Check sheet for the modelled part. Datum: model origin and axes. Units: mm. Give positions to 0.01 mm unless a question says otherwise; leave off trailing zeros. Loops run counter-clockwise (first coordinate to the right, second up) from the corner with the lowest first, then second, coordinate; pieces in that order, holes last. Notation, with made-up numbers: (-8.75, 55.5) -> (22.25, 55.5) arc R18 cw to (22.25, 68.5) -> close; hole circle Ø10 at (20.5, 16). An arc over 180 degrees is marked (long way). Write each question's results on one line, items separated by ' | '. Start each with the question number.
1. Cross-section at B-B on y = 4. Record the boundary of the cut face in (x, z), and give its area (3 significant figures).
2. Cross-section at D-D on z = 2.1. Count the separate pieces of the cut face and the enclosed holes in it, and give its area (3 significant figures).
3. Cross-section at A-A on x = -0.5. Record the boundary of the cut face in (y, z).
4. Cross-section at C-C on x = -48. Record the boundary of the cut face in (y, z), and give its area (3 significant figures).
5. Gauge pin test, flat ends, axial feed: pin 1 Ø2.5 at (x, z) = (-18, 3) entering from +Y; pin 2 Ø3 at (y, z) = (18.5, 0.5) entering from -X; pin 3 Ø2.5 at (x, z) = (-105.5, 3) entering from +Y; pin 4 Ø4.5 at (x, y) = (51.5, 4) entering from +Z. Record the tip position at first contact, or that the pin passes through.
6. Material ranges on L1, parallel to Y at x = 25.5, z = 3.75; L2, parallel to Y at x = -27.5, z = 2.1; L3, parallel to X at y = 48, z = 2.8, recorded low to high. Write a range as from..to.
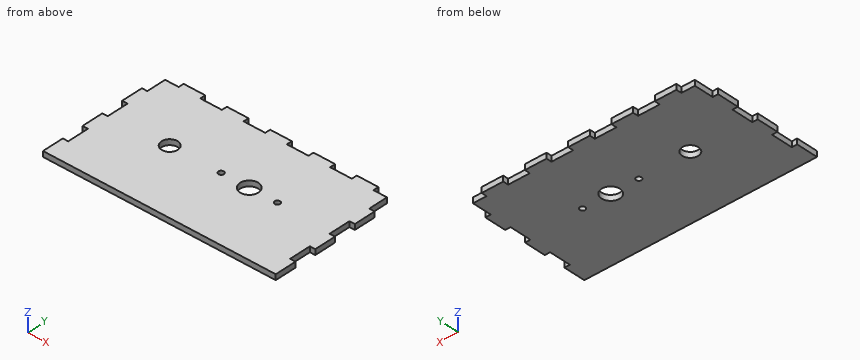
from build123d import *

# Parameters (mm, degrees)
SKETCH_1_W               = 205
SKETCH_1_H               = 118
SKETCH_1_R               = 8.5
SKETCH_1_R_2             = 7.5
SKETCH_1_R_3             = 2.5
EXTRUDE_1_DEPTH          = 5
SKETCH_2_W               = 5
SKETCH_2_H               = 20
EXTRUDE_2_DEPTH          = 5
PATTERN_LINEAR_2_COUNT   = 3
PATTERN_LINEAR_2_PITCH   = 40
MIRROR_2_COPY_1_SKETCH_W = 5
MIRROR_2_COPY_1_SKETCH_H = 20
MIRROR_2_COPY_1_DEPTH    = 5
MIRROR_2_COPY_2_SKETCH_W = 5
MIRROR_2_COPY_2_SKETCH_H = 20
MIRROR_2_COPY_2_DEPTH    = 5
SKETCH_3_W               = 20
SKETCH_3_H               = 5
EXTRUDE_3_DEPTH          = 5
PATTERN_LINEAR_3_COUNT   = 3
PATTERN_LINEAR_3_PITCH   = 40
PATTERN_LINEAR_4_COUNT   = 3
PATTERN_LINEAR_4_PITCH   = 40


with BuildPart() as part:
    # 스케치1 → 보스-돌출1 (new body)
    with BuildSketch(Plane.XY):
        Rectangle(SKETCH_1_W, SKETCH_1_H)
        with Locations((25.5, 4)):
            Circle(SKETCH_1_R, mode=Mode.SUBTRACT)
        with Locations((-48, 4)):
            Circle(SKETCH_1_R_2, mode=Mode.SUBTRACT)
        with Locations((-0.5, 4)):
            Circle(SKETCH_1_R_3, mode=Mode.SUBTRACT)
        with Locations((51.5, 4)):
            Circle(SKETCH_1_R_3, mode=Mode.SUBTRACT)
    extrude(amount=EXTRUDE_1_DEPTH)

    # 스케치2 → 보스-돌출2 (add)
    with BuildSketch(Plane.XY.offset(5)):
        with Locations((105, -49)):
            Rectangle(SKETCH_2_W, SKETCH_2_H)
    extrude_2 = extrude(amount=-EXTRUDE_2_DEPTH)

    # 선형 패턴2: 보스-돌출2 ×3
    with Locations(*[(0, i * PATTERN_LINEAR_2_PITCH, 0) for i in range(1, PATTERN_LINEAR_2_COUNT)]):
        add(extrude_2)

    # 대칭 복사2: 보스-돌출2 across plane
    add(extrude_2.mirror(Plane(origin=(0, 0, 0), x_dir=(0, 0, 1), z_dir=(1, 0, 0))))

    # 대칭 복사2 copy 1 sketch → 대칭 복사2 copy 1 (add)
    with BuildSketch(Plane(origin=(0, 40, 5), x_dir=(-1, 0, 0), z_dir=(0, 0, 1))):
        with Locations((105, 49)):
            Rectangle(MIRROR_2_COPY_1_SKETCH_W, MIRROR_2_COPY_1_SKETCH_H)
    extrude(amount=-MIRROR_2_COPY_1_DEPTH)

    # 대칭 복사2 copy 2 sketch → 대칭 복사2 copy 2 (add)
    with BuildSketch(Plane(origin=(0, 80, 5), x_dir=(-1, 0, 0), z_dir=(0, 0, 1))):
        with Locations((105, 49)):
            Rectangle(MIRROR_2_COPY_2_SKETCH_W, MIRROR_2_COPY_2_SKETCH_H)
    extrude(amount=-MIRROR_2_COPY_2_DEPTH)

    # 스케치3 → 보스-돌출3 (add)
    with BuildSketch(Plane.XY.offset(5)):
        with Locations((0, 61.5)):
            Rectangle(SKETCH_3_W, SKETCH_3_H)
    extrude_3 = extrude(amount=-EXTRUDE_3_DEPTH)

    # 선형 패턴3: 보스-돌출3 ×3
    with Locations(*[(i * PATTERN_LINEAR_3_PITCH, 0, 0) for i in range(1, PATTERN_LINEAR_3_COUNT)]):
        add(extrude_3)

    # 선형 패턴4: 보스-돌출3 ×3
    with Locations(*[(-i * PATTERN_LINEAR_4_PITCH, 0, 0) for i in range(1, PATTERN_LINEAR_4_COUNT)]):
        add(extrude_3)


solid = part.part
Geometry says:
1) outline: (-102.5, 0) -> (-55.5, 0) -> (-55.5, 5) -> (-102.5, 5) -> close; (-40.5, 0) -> (-3, 0) -> (-3, 5) -> (-40.5, 5) -> close; (2, 0) -> (17, 0) -> (17, 5) -> (2, 5) -> close; (34, 0) -> (49, 0) -> (49, 5) -> (34, 5) -> close; (54, 0) -> (102.5, 0) -> (102.5, 5) -> (54, 5) -> close | area: 815 mm^2
2) separate pieces: 1 | enclosed holes: 4 | area: 24,800 mm^2
3) outline: (-59, 0) -> (1.5, 0) -> (1.5, 5) -> (-59, 5) -> close; (6.5, 0) -> (64, 0) -> (64, 5) -> (6.5, 5) -> close
4) outline: (-59, 0) -> (-3.5, 0) -> (-3.5, 5) -> (-59, 5) -> close; (11.5, 0) -> (64, 0) -> (64, 5) -> (11.5, 5) -> close | area: 540 mm^2
5) pin 1: y = 59 | pin 2: x = -102.5 | pin 3: y = 41 | pin 4: through
6) L1: -59..-4.5, 12.5..59 | L2: -59..59 | L3: -102.5..102.5
